Autodesk Inventor part; units mm, degrees
ref_plane "YZ Plane" through (0, 0, 0) normal (1, 0, 0) x (0, 1, 0)
ref_plane "XZ Plane" through (0, 0, 0) normal (0, 1, 0) x (-1, 0, 0)
ref_plane "XY Plane" through (0, 0, 0) normal (0, 0, 1) x (1, 0, 0)
sketch "Sketch1" plane through (0, 0, 0) normal (0, 1, 0) x (-1, 0, 0)
  line L0 (-27, 15) -> (27, 15)
  line L1 (30, 12) -> (30, -12)
  line L2 (27, -15) -> (-27, -15)
  line L3 (-30, -12) -> (-30, 12)
  line L4 (-30, 15) -> (30, -15) construction
  line L5 (30, 15) -> (-30, -15) construction
  arc A0 (30, 12) -> (27, 15) centre (27, 12) ccw
  arc A1 (27, -15) -> (30, -12) centre (27, -12) ccw
  arc A2 (-30, -12) -> (-27, -15) centre (-27, -12) ccw
  arc A3 (-27, 15) -> (-30, 12) centre (-27, 12) ccw
  line L6 (28, -12) -> (28, 12)
  arc A4 (28, 12) -> (27, 13) centre (27, 12) ccw
  line L7 (27, 13) -> (-27, 13)
  arc A5 (-27, 13) -> (-28, 12) centre (-27, 12) ccw
  line L8 (-28, 12) -> (-28, -12)
  arc A6 (-28, -12) -> (-27, -13) centre (-27, -12) ccw
  line L9 (-27, -13) -> (27, -13)
  arc A7 (27, -13) -> (28, -12) centre (27, -12) ccw
  line L10 (-26, -4) -> (-30, -4)
  line L11 (-30, -4) -> (-30, 4)
  line L12 (-30, 4) -> (-26, 4)
  line L13 (-26, 4) -> (-26, -4)
  line L14 (-26, -4) -> (-30, 4) construction
  line L15 (-30, -4) -> (-26, 4) construction
  point P0 (0, 0)
  point P1 (-28, 0)
  point P2 (-28, 4)
  point P3 (-28, -4)
  dimension "d0" = 30
  dimension "d1" = 60
  dimension "d2" = 3
  dimension "d3" = 3
  dimension "d4" = 2
  dimension "d7" = 8
extrude "Extrusion1" add sketch "Sketch1" along normal blind 2 contours L0 A0 L1 A1 L2 A2 L3 L10 L8 A6 L9 A7 L6 A4 L7 A5 L12 A3 | L12 L8 L10 L3 | L12 L13 L10 L8
sketch "Sketch2" plane through (0, 2, 0) normal (0, 1, 0) x (1, 0, 0)
  line L0 (26, -4) -> (28, -4)
  line L1 (34, 4) -> (26, 4)
  line L2 (26, 4) -> (26, -4)
  line L3 (26, -4) -> (34, -4)
  line L4 (34, -4) -> (34, 4)
  line L5 (30, -12) -> (30, 12)
  line L6 (34, 4) -> (26, -4) construction
  line L7 (26, 4) -> (34, -4) construction
  point P0 (0, 0)
  point P1 (30, 0)
extrude "Extrusion2" add sketch "Sketch2" along normal blind 2
fillet "Fillet1" radius 2 3 edges at (26, 4, 0) (30, 4, -4) (30, 4, 4)
fillet "Fillet2" radius 2 2 edges at (28, 1, -4) (28, 1, 4)
properties part number "SolarpanelAdapter_bot" material "ABS Plastic"
Source: CAD feature listing. Evaluate the final solid. Frame: model axes, mm. A direction names the side the tool comes from. Coordinates: 2 decimals unless noted, no trailing zeros. Loops run counter-clockwise (first coordinate to the right, second up) from the corner with the lowest first, then second, coordinate; pieces in that order, holes last. Notation, with made-up numbers: (3.25, 42) - (56.25, 42) arc R23 cw to (56.25, 80) - close; hole circle Ø10 at (-38, 75.5). An arc over 180 degrees is marked (long way). Answer as CSV lines item,"result".
1. Reachability of faces 1 (the flat face through (0, 1, -13)), 2 (the flat face through (30, 1, 0)), 3 (the cylindrical face through (26.4, 3.2, 0.1)) from +Z, -Z, +X, -X, +Y, -Y: full face, straight path, thin tool, end or side. Return the list, or none.
Established:
face 1,"+Y, -Y"
face 2,"+Z, -Z, +X, -Y"
face 3,"+Z, -Z, -X, +Y"
2. Section A-A (z = 7.75). Return loops of the section in (x, y).
Established:
outline,"(-30, 0) - (-28, 0) - (-28, 2) - (-30, 2) - close; (28, 0) - (30, 0) - (30, 2) - (28, 2) - close"
3. Contact query for flat-ended pins moving along their axis: pin 1 (4.5 mm diameter, centred on x = 32.5, z = -1, fed in from -Y); pin 2 (1 mm diameter, centred on x = 31, y = 1, fed in from +Z); pin 3 (0.6 mm diameter, centred on y = 1, z = -0.5, fed in from +X). Output: stop coordinate, or through.
Established:
pin 1,"stops at y = 2"
pin 2,"passes through"
pin 3,"stops at x = 30"
4. Mould query, pull axis Z, two halves, no side actions, for faces 4 (the cylindrical face through (29.94, 3.4, 3.43)), 5 (the flat face through (31, 4, 0)), 6 (the flat face through (-28, 1, 0)), 7 (the cylindrical face through (27.43, 1.01, 4.6)). Classes: released by +Z, released by -Z, zero draft, split by the parting line, or undercut.
Established:
face 4,"released by +Z"
face 5,"zero draft"
face 6,"undercut"
face 7,"undercut"
5. Ray query, line 1 (Z direction, x = -1.5, y = 1.6); line 2 (X direction, y = 0.45, z = -7.25); line 3 (X direction, y = 1.5, z = -0.5). Return the intervals inside material, ascending.
Established:
line 1,"z = -15 to -13, 13 to 15"
line 2,"x = -30 to -28, 28 to 30"
line 3,"x = -30 to -28, 26 to 30"
6. Section B-B (x = -1.5). Return loops of the section in (y, z), then the cut area to 3 significant figures.
Established:
outline,"(0, -15) - (2, -15) - (2, -13) - (0, -13) - close; (0, 13) - (2, 13) - (2, 15) - (0, 15) - close"
area,"8.00 mm2"
